from build123d import *

# Parameters (mm, degrees)
ESBO_O1_W                = 190
ESBO_O1_H                = 190
RESSALTO_EXTRUS_O1_DEPTH = 5
FILETE1_R                = 35
ESBO_O2_R                = 1
CORTE_EXTRUS_O1_DEPTH    = 135.443296597
CORTE_EXTRUS_O2_DEPTH    = 10
SKETCH3_R                = 1.25
CUT_EXTRUDE1_DEPTH       = 135.443296597
SKETCH5_R                = 1
CUT_EXTRUDE3_DEPTH       = 135.443296597
SKETCH7_W                = 13.35
SKETCH7_H                = 8.4
CUT_EXTRUDE5_DEPTH       = 135.443296597
CUT_EXTRUDE6_DEPTH       = 135.443296597


with BuildPart() as part:
    # Esboço1 → Ressalto-extrusão1 (new body)
    with BuildSketch(Plane(origin=(0, 0, 0), x_dir=(1, 0, 0), z_dir=(0, 1, 0))):
        Rectangle(ESBO_O1_W, ESBO_O1_H)
    extrude(amount=RESSALTO_EXTRUS_O1_DEPTH)

    # Filete1
    filete1_edges = [part.edges().sort_by_distance(p)[0] for p in [
        (95, 2.5, 95),
        (-95, 2.5, 95),
        (-95, 2.5, -95),
        (95, 2.5, -95),
    ]]
    fillet(filete1_edges, radius=FILETE1_R)

    # Esboço2 → Corte-extrusão1 (cut, through all)
    with BuildSketch(Plane(origin=(0, 5, 0), x_dir=(1, 0, 0), z_dir=(0, 1, 0))):
        with Locations(Location((-55, 90, 0), (0, 0, 270))):
            Circle(ESBO_O2_R)
        with Locations(Location((55, 90, 0), (0, 0, 90))):
            Circle(ESBO_O2_R)
        with Locations(Location((55, -90, 0), (0, 0, 270))):
            Circle(ESBO_O2_R)
        with Locations(Location((-55, -90, 0), (0, 0, 90))):
            Circle(ESBO_O2_R)
    extrude(amount=-CORTE_EXTRUS_O1_DEPTH, mode=Mode.SUBTRACT)

    # Esboço3 → Corte-extrusão2 (cut)
    with BuildSketch(Plane(origin=(0, 5, 0), x_dir=(1, 0, 0), z_dir=(0, 1, 0))):
        with BuildLine():
            Line((-60, 39.5), (60, 39.5))
            ThreePointArc((60, 39.5), (61.414213562, 38.914213562), (62, 37.5))
            Line((62, 37.5), (62, -37.5))
            ThreePointArc((62, -37.5), (61.414213562, -38.914213562), (60, -39.5))
            Line((60, -39.5), (-60, -39.5))
            ThreePointArc((-60, -39.5), (-61.414213562, -38.914213562), (-62, -37.5))
            Line((-62, -37.5), (-62, 37.5))
            ThreePointArc((-62, 37.5), (-61.414213562, 38.914213562), (-60, 39.5))
        make_face()
    extrude(amount=-CORTE_EXTRUS_O2_DEPTH, mode=Mode.SUBTRACT)

    # Sketch3 → Cut-Extrude1 (cut, through all)
    with BuildSketch(Plane(origin=(0, 5, 0), x_dir=(1, 0, 0), z_dir=(0, 1, 0))):
        with Locations(Location((22.50310845, 47.5, 0), (0, 0, 270))):
            Circle(SKETCH3_R)
        with Locations(Location((-22.49689155, 47.5, 0), (0, 0, 270))):
            Circle(SKETCH3_R)
        with Locations(Location((-11.39689155, 72.5, 0), (0, 0, 270))):
            Circle(SKETCH3_R)
        with Locations(Location((11.40310845, 72.5, 0), (0, 0, 270))):
            Circle(SKETCH3_R)
        with Locations(Location((11.40310845, -72.5, 0), (0, 0, 90))):
            Circle(SKETCH3_R)
        with Locations(Location((-11.39689155, -72.5, 0), (0, 0, 90))):
            Circle(SKETCH3_R)
        with Locations(Location((-22.49689155, -47.5, 0), (0, 0, 90))):
            Circle(SKETCH3_R)
        with Locations(Location((22.50310845, -47.5, 0), (0, 0, 90))):
            Circle(SKETCH3_R)
    extrude(amount=-CUT_EXTRUDE1_DEPTH, mode=Mode.SUBTRACT)

    # Sketch5 → Cut-Extrude3 (cut, through all)
    with BuildSketch(Plane(origin=(0, 5, 0), x_dir=(1, 0, 0), z_dir=(0, 1, 0))):
        with Locations(Location((87.705642178, 46.088474581, 0), (0, 0, 270))):
            Circle(SKETCH5_R)
        with Locations(Location((87.705642178, 39.070544877, 0), (0, 0, 270))):
            Circle(SKETCH5_R)
    extrude(amount=-CUT_EXTRUDE3_DEPTH, mode=Mode.SUBTRACT)

    # Sketch7 → Cut-Extrude5 (cut, through all)
    with BuildSketch(Plane(origin=(0, 5, 0), x_dir=(1, 0, 0), z_dir=(0, 1, 0))):
        with Locations((37.711300079, 85.8)):
            Rectangle(SKETCH7_W, SKETCH7_H)
    extrude(amount=-CUT_EXTRUDE5_DEPTH, mode=Mode.SUBTRACT)

    # Sketch8 → Cut-Extrude6 (cut, through all)
    with BuildSketch(Plane(origin=(0, 5, 0), x_dir=(1, 0, 0), z_dir=(0, 1, 0))):
        with BuildLine():
            Line((6.00310845, -50), (-5.99689155, -50))
            ThreePointArc((-5.99689155, -50), (-7.057551722, -49.560660172), (-7.49689155, -48.5))
            Line((-7.49689155, -48.5), (-7.49689155, -44))
            ThreePointArc((-7.49689155, -44), (-7.057551722, -42.939339828), (-5.99689155, -42.5))
            Line((-5.99689155, -42.5), (6.00310845, -42.5))
            ThreePointArc((6.00310845, -42.5), (7.063768622, -42.939339828), (7.50310845, -44))
            Line((7.50310845, -44), (7.50310845, -48.5))
            ThreePointArc((7.50310845, -48.5), (7.063768622, -49.560660172), (6.00310845, -50))
        make_face()
        with BuildLine():
            Line((-7.49689155, 48.5), (-7.49689155, 44))
            ThreePointArc((-7.49689155, 44), (-7.057551722, 42.939339828), (-5.99689155, 42.5))
            Line((-5.99689155, 42.5), (6.00310845, 42.5))
            ThreePointArc((6.00310845, 42.5), (7.063768622, 42.939339828), (7.50310845, 44))
            Line((7.50310845, 44), (7.50310845, 48.5))
            ThreePointArc((7.50310845, 48.5), (7.063768622, 49.560660172), (6.00310845, 50))
            Line((6.00310845, 50), (-5.99689155, 50))
            ThreePointArc((-5.99689155, 50), (-7.057551722, 49.560660172), (-7.49689155, 48.5))
        make_face()
    extrude(amount=-CUT_EXTRUDE6_DEPTH, mode=Mode.SUBTRACT)


solid = part.part
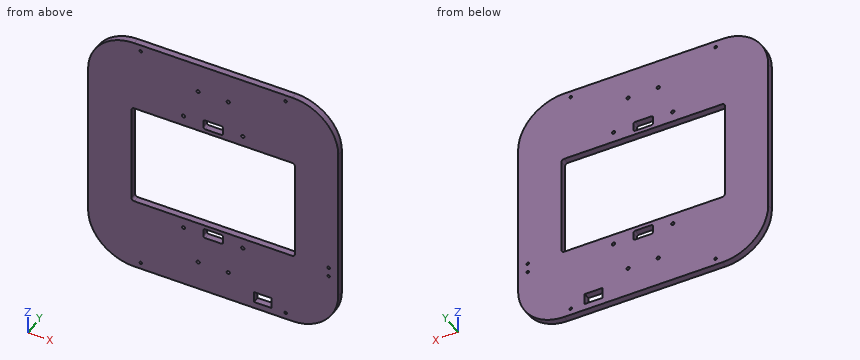
CAD build for the part. Positions are in the model's coordinates, mm. Coordinates: 2 decimals unless noted, no trailing zeros. Write each loop counter-clockwise with the first axis right and the second up, starting at its lowest first coordinate (ties: lowest second). Pieces come first, ordered by that corner, then holes. Notation, with made-up numbers: M 83.25,-9.75 L 102.25,-9.75 A10 ccw 102.25,-4.75 Z; hole C 82.5,50.5 d6. An arc over 180 degrees is marked long. Answer as a JSON object with one key per item and string values. Group by question number.
1) Pin check, flat tip, straight feed: pin 1 Ø1.5 at (y, z) = (3, -84.5) entering from +X. Stop position of the tip, or through.
2) Saw through at C-C (z = 29). Write the cut outline in (x, y), plus the area to 3 significant figures.
3) Wall check: line 1 (X direction, y = 2.3, z = -47.5); line 2 (Z direction, x = 31.5, y = 3.05); line 3 (Z direction, x = -22.5, y = 1.3). Give the ranges that are in metal, low to high. Write a range as from..to.
4) Saw through at D-D (y = 3.65). Give the number of separate pieces and of enclosed holes in the cut face, plus the area to 3 significant figures.
5) Saw through at B-B (x = 41). Write the cut outline in (y, z), plus the area to 3 significant figures.
6) Saw through at A-A (x = -35). Write the cut outline in (y, z).
Values follow:
{
 "1": {"pin 1": "stops at x = 85.71"},
 "2": {"outline": "M -95,0 L -62,0 L -62,5 L -95,5 Z; M 62,0 L 95,0 L 95,5 L 62,5 Z", "area": "330 mm2"},
 "3": {"line 1": "x = -95..-23.75, -21.25..-7.5, 7.5..21.25, 23.75..95", "line 2": "z = -95..-90, -81.6..-39.5, 39.5..95", "line 3": "z = -95..-48.75, -46.25..-39.5, 39.5..46.25, 48.75..95"},
 "4": {"separate pieces": "1", "enclosed holes": "18", "area": "24,900 mm2"},
 "5": {"outline": "M 0,-95 L 5,-95 L 5,-90 L 0,-90 Z; M 0,-81.6 L 5,-81.6 L 5,-39.5 L 0,-39.5 Z; M 0,39.5 L 5,39.5 L 5,95 L 0,95 Z", "area": "513 mm2"},
 "6": {"outline": "M 0,-95 L 5,-95 L 5,-39.5 L 0,-39.5 Z; M 0,39.5 L 5,39.5 L 5,95 L 0,95 Z"}
}
